Geometry: final body of the model. Coordinates: model frame, mm. A direction names the side the tool comes from. Coordinates: 2 decimals unless noted, no trailing zeros. Write each loop counter-clockwise with the first axis right and the second up, starting at its lowest first coordinate (ties: lowest second). Pieces come first, ordered by that corner, then holes. Notation, with made-up numbers: (31, -17.5) - (47, -17.5) arc R22 cw to (47, -11.5) - close; hole circle Ø8 at (86.5, 33). An arc over 180 degrees is marked (long way). Answer as a JSON object with one key per item and string values. Group by question number.
Item 1: Set-up query: faces 1 (the flat face through (105, 0, -42)), 2 (the flat face through (10, -0.6, -47.3)), 3 (the flat face through (105, -0.81, -42)), 4 (the flat face through (202, -0.6, -47.3)). Return all of +Z, -Z, +X, -X, +Y, -Y with unobstructed straight access to the full face (end or side cutting, diameter ignored); none if empty.
Item 2: Section A-A on x = 104. Return loops of the section in (y, z).
Item 3: First-contact query: pin 1 Ø1.5 at (x, z) = (161, -72) entering from +Y; pin 2 Ø4 at (x, y) = (166, 2.5) entering from +Z. Flat tips, straight axial feed; report the tip coordinate or a pass-through.
Item 4: Line query: line 1 along Y through (x, z) = (189.5, -59); line 2 along Z through (x, y) = (57.5, 7.25). Output: solid intervals per line, ascending. Write a range as from..to.
Item 5: Section C-C on z = -65.5. Return loops of the section in (x, y), and give its area (3 significant figures).
Item 6: Section B-B on y = 4. Return loops of the section in (x, z), and give its area (3 significant figures).
```python
from build123d import *

# Parameters (mm, degrees)
SKETCH1_W                    = 212
SKETCH1_H                    = 85
BASE_FLANGE1_DEPTH           = 0.81
CUT_EXTRUDE1_REACH           = 230.407
SKETCH6_W                    = 10
SKETCH6_H                    = 75
EDGE_FLANGE1_STRIP_W         = 4.7132
EDGE_FLANGE1_STRIP_H         = 0.81
EDGE_FLANGE1_STRIP_CUT_DEPTH = 192
EDGE_FLANGE1_DEPTH           = 192


# Sheet-metal steps are written as plain solids
with BuildPart() as part:
    # Sketch1 → Base-Flange1 (new body)
    with BuildSketch(Plane(origin=(0, 0, 0), x_dir=(1, 0, 0), z_dir=(0, 1, 0))):
        with Locations((106, 42.5)):
            Rectangle(SKETCH1_W, SKETCH1_H)
    extrude(amount=-BASE_FLANGE1_DEPTH)

    # Sketch6 → Cut-Extrude1 (cut, up to next)
    with BuildSketch(Plane(origin=(0, 0, 0), x_dir=(1, 0, 0), z_dir=(0, 1, 0)), mode=Mode.PRIVATE) as cut_extrude1_sk1:
        with Locations((5, 47.5)):
            Rectangle(SKETCH6_W, SKETCH6_H)
    cut_extrude1_tool1 = extrude(cut_extrude1_sk1.sketch, amount=-CUT_EXTRUDE1_REACH, mode=Mode.PRIVATE) & part.part
    # Sketch6 → Cut-Extrude1 (cut, up to next)
    with BuildSketch(Plane(origin=(0, 0, 0), x_dir=(1, 0, 0), z_dir=(0, 1, 0)), mode=Mode.PRIVATE) as cut_extrude1_sk2:
        with Locations((207, 47.5)):
            Rectangle(SKETCH6_W, SKETCH6_H)
    cut_extrude1_tool2 = extrude(cut_extrude1_sk2.sketch, amount=-CUT_EXTRUDE1_REACH, mode=Mode.PRIVATE) & part.part
    add(cut_extrude1_tool1.solids().sort_by_distance((5, 0, -47.5))[0], mode=Mode.SUBTRACT)
    add(cut_extrude1_tool2.solids().sort_by_distance((207, 0, -47.5))[0], mode=Mode.SUBTRACT)

    # Edge-Flange1 strip (across the edge) → Edge-Flange1 strip cut (cut)
    with BuildSketch(Plane(origin=(202, 0, -85), x_dir=(0, 0, 1), z_dir=(-1, 0, 0))):
        with Locations((-0.81, -0.405)):
            Rectangle(EDGE_FLANGE1_STRIP_W, EDGE_FLANGE1_STRIP_H)
    extrude(amount=EDGE_FLANGE1_STRIP_CUT_DEPTH, mode=Mode.SUBTRACT)

    # Edge-Flange1 section (across the edge) → Edge-Flange1 (add)
    with BuildSketch(Plane(origin=(202, 0, -85), x_dir=(0, 0, 1), z_dir=(-1, 0, 0))):
        with BuildLine():
            Line((0, 0.7366), (0, 8))
            Line((0, 8), (0.81, 8))
            Line((0.81, 8), (0.81, 0.7366))
            ThreePointArc((0.81, 0.7366), (1.025745145, 0.215745145), (1.5466, 0))
            Line((1.5466, 0), (1.5466, -0.81))
            ThreePointArc((1.5466, -0.81), (0.452988652, -0.357011348), (0, 0.7366))
        make_face()
    extrude(amount=EDGE_FLANGE1_DEPTH)


solid = part.part
```
Checks:
{
 "1": {"face 1": "+Z, +X, -X, +Y", "face 2": "-Z, -X, +Y, -Y", "face 3": "+Z, -Z, +X, -X, -Y", "face 4": "-Z, +X, +Y, -Y"},
 "2": {"outline": "(-0.81, -83.45) arc R1.55 ccw to (0.74, -85) - (8, -85) - (8, -84.19) - (0.74, -84.19) arc R0.74 cw to (0, -83.45) - (0, 0) - (-0.81, 0) - close"},
 "3": {"pin 1": "y = 0", "pin 2": "z = -84.15"},
 "4": {"line 1": "-0.81..0", "line 2": "-85..-84.19"},
 "5": {"outline": "(10, -0.81) - (202, -0.81) - (202, 0) - (10, 0) - close", "area": "156 mm^2"},
 "6": {"outline": "(10, -85) - (202, -85) - (202, -84.19) - (10, -84.19) - close", "area": "156 mm^2"}
}
